Print and shaded views of the part. All mm, measured from the part's lowest x, y and z. A direction names the side the tool comes from. Round coordinates to 2 decimals unless told otherwise and drop trailing zeros. Order: outer loops, then holes, each group sorted by start corner. A loop starts at its lowest first (then second) coordinate and runs counter-clockwise, first axis right, second up. Notation, with made-up numbers: (44.25, 50) - (91.25, 50) arc R29 ccw to (91.25, 82) - close; hole circle Ø11 at (-11, -3.75). An arc over 180 degrees is marked (long way). Return JSON: item names as keys, results as strings. Group by question number.
Item 1: Two-plate mould, pull along Z, no slides. Class the marked faces 3, 4 and 5: released by +Z, released by -Z, zero draft, split by the parting line, or undercut.
Item 2: Drop flat-ended pins along their axis: pin 1 (3 mm diameter, centred on x = 4.5, z = 3, fed in from +Y); pin 2 (4.5 mm diameter, centred on x = 5.5, z = 5.5, fed in from +Y); pin 3 (2 mm diameter, centred on x = 9, y = 3.5, fed in from +Z). Give the stop position or say it passes through.
Item 3: Saw through at B-B on y = 1.65. List the corners of the cut face in (x, z).
Item 4: Tool access for the marked faces 1 and 2: list every direction of +Z, -Z, +X, -X, +Y, -Y with a clear straight run to the whole face (end or side of a thin tool).
Item 5: Saw through at C-C on x = 5.5. List the corners of the cut face in (y, z).
Item 6: Saw through at A-A on z = 13.5. List the corners of the cut face in (x, y), and give its area (3 significant figures).
Item 7: Saw through at D-D on y = 3.1. List the corners of the cut face in (x, z).
Item 8: Probe probe 1 along Z at (x, y) = (5.5, 0.9); probe 2 along X at (y, z) = (4.6, 13.5); probe 3 along X at (y, z) = (0.75, 5.5). List the from-to ranges inside material, lowest first.
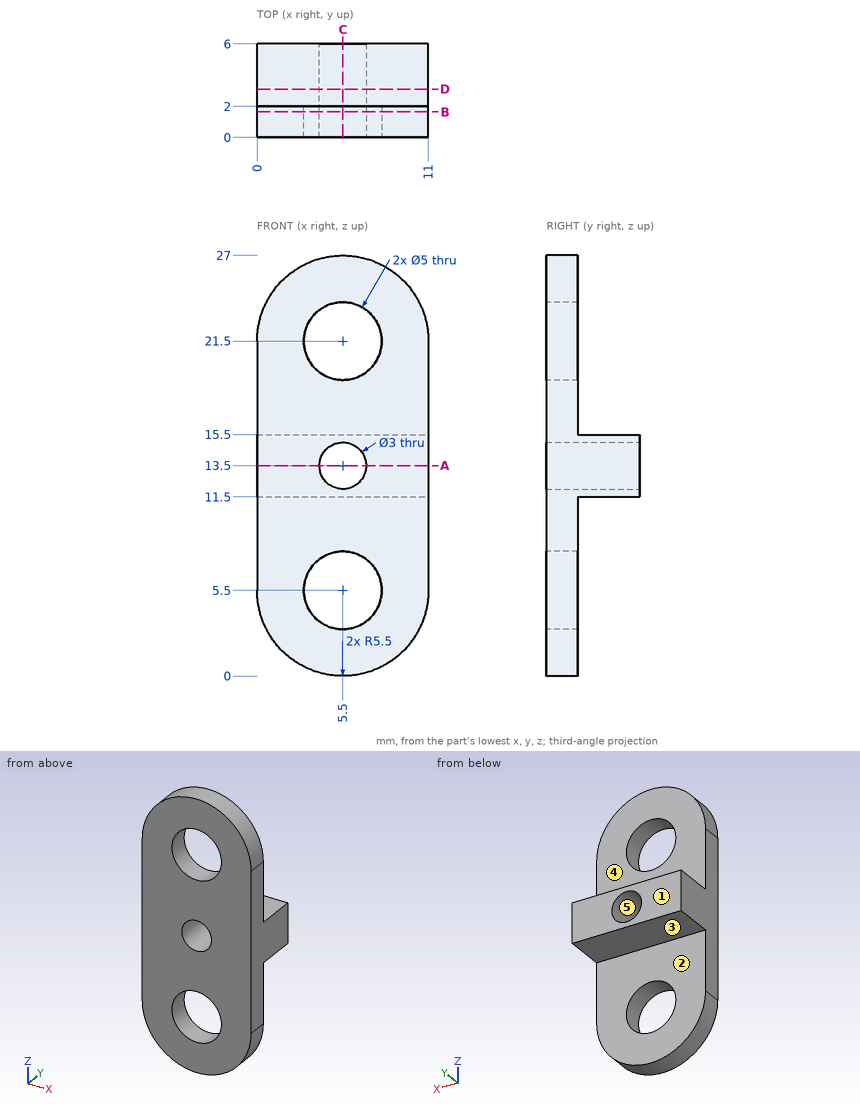
Filled in:
{
 "1": {"face 3": "released by -Z", "face 4": "zero draft", "face 5": "undercut"},
 "2": {"pin 1": "stops at y = 2", "pin 2": "passes through", "pin 3": "stops at z = 15.5"},
 "3": {"outline": "(0, 5.5) arc R5.5 ccw to (11, 5.5) - (11, 21.5) arc R5.5 ccw to (0, 21.5) - close; hole circle Ø5 at (5.5, 5.5); hole circle Ø5 at (5.5, 21.5); hole circle Ø3 at (5.5, 13.5)"},
 "4": {"face 1": "+Z, -Z, +X, -X, +Y", "face 2": "-Z, +X, -X, +Y"},
 "5": {"outline": "(0, 0) - (2, 0) - (2, 3) - (0, 3) - close; (0, 8) - (2, 8) - (2, 11.5) - (6, 11.5) - (6, 12) - (0, 12) - close; (0, 15) - (6, 15) - (6, 15.5) - (2, 15.5) - (2, 19) - (0, 19) - close; (0, 24) - (2, 24) - (2, 27) - (0, 27) - close"},
 "6": {"outline": "(0, 0) - (4, 0) - (4, 6) - (0, 6) - close; (7, 0) - (11, 0) - (11, 6) - (7, 6) - close", "area": "48.0 mm^2"},
 "7": {"outline": "(0, 11.5) - (11, 11.5) - (11, 15.5) - (0, 15.5) - close; hole circle Ø3 at (5.5, 13.5)"},
 "8": {"probe 1": "z = 0 to 3, 8 to 12, 15 to 19, 24 to 27", "probe 2": "x = 0 to 4, 7 to 11", "probe 3": "x = 0 to 3, 8 to 11"}
}
